```python
from build123d import *

# Parameters (mm, degrees)
F1_DEPTH  = 20
F3_DEPTH  = 25
F6_DEPTH  = 4
F8_R      = 1.395
F9_DEPTH  = 1.5
F8_R_2    = 4.25
F10_DEPTH = 112.584302492
F8_R_3    = 5.5
F11_DEPTH = 2


with BuildPart() as f1:
    # F0 (on Front) → F1 (new body)
    with BuildSketch(Plane.XZ):
        with BuildLine():
            Line((-35, 51.9615242271), (-65, 0))
            Line((-65, 0), (65, 0))
            Line((65, 0), (65, 10))
            Line((65, 10), (20.0384757729, 10))
            ThreePointArc((20.0384757729, 10), (14.8620948709, 10.6814834742), (10.0384757729, 12.6794919243))
            Line((10.0384757729, 12.6794919243), (-3.5109076373, 20.5022320835))
            ThreePointArc((-3.5109076373, 20.5022320835), (-4.2097963767, 21.4130416216), (-4.0599457429, 22.5512701892))
            Line((-4.0599457429, 22.5512701892), (-3.5599457429, 23.417295593))
            Line((-3.5599457429, 23.417295593), (-20.8804538186, 33.417295593))
            Line((-20.8804538186, 33.417295593), (-21.3804538186, 32.5512701892))
            ThreePointArc((-21.3804538186, 32.5512701892), (-22.2912633567, 31.8523814498), (-23.4294919243, 32.0022320835))
            Line((-23.4294919243, 32.0022320835), (-38.1519237886, 40.5022320835))
            ThreePointArc((-38.1519237886, 40.5022320835), (-38.8508125281, 41.4130416216), (-38.7009618943, 42.5512701892))
            Line((-38.7009618943, 42.5512701892), (-33.7009618943, 51.2115242271))
            Line((-33.7009618943, 51.2115242271), (-35, 51.9615242271))
        make_face()
        with BuildLine():
            ThreePointArc((-52.6208348754, 8.4413429511), (-54.9504640068, 11.4773747445), (-54.4509618943, 15.27146997))
            Line((-54.4509618943, 15.27146997), (-42.7009618943, 35.6230669589))
            ThreePointArc((-42.7009618943, 35.6230669589), (-39.6649301009, 37.9526960904), (-35.8708348754, 37.4531939779))
            Line((-35.8708348754, 37.4531939779), (10.2416697508, 10.8301270189))
            ThreePointArc((10.2416697508, 10.8301270189), (12.5712988822, 5.2059047745), (7.7416697508, 1.5))
            Line((7.7416697508, 1.5), (-40.5980762114, 1.5))
            Line((-40.5980762114, 1.5), (-52.6208348754, 8.4413429511))
        make_face(mode=Mode.SUBTRACT)
    extrude(amount=F1_DEPTH)

    # F2 (on face) → F3 (cut)
    with BuildSketch(Plane.XY.offset(10)):
        with BuildLine():
            Line((65, -17.963156903), (65, -15))
            Line((65, -15), (33, -15))
            ThreePointArc((33, -15), (30.8786796564, -15.8786796564), (30, -18))
            Line((30, -18), (30, -20))
            Line((30, -20), (65, -20))
            Line((65, -20), (65, -17.963156903))
        make_face()
        with BuildLine():
            Line((65, -7), (48, -7))
            ThreePointArc((48, -7), (45, -10), (48, -13))
            Line((48, -13), (65, -13))
            Line((65, -13), (65, -7))
        make_face()
        with BuildLine():
            Line((33, -5), (65, -5))
            Line((65, -5), (65, -2.036843097))
            Line((65, -2.036843097), (65, 0))
            Line((65, 0), (30, 0))
            Line((30, 0), (30, -2))
            ThreePointArc((30, -2), (30.8786796564, -4.1213203436), (33, -5))
        make_face()
    extrude(amount=-F3_DEPTH, mode=Mode.SUBTRACT)

    # F5 (on offset) → F6 (cut, through all)
    with BuildSketch(Plane(origin=(9.25, 0, 16.02146997), x_dir=(0.8660254038, 0, -0.5), z_dir=(0.5, 0, 0.8660254038))):
        with BuildLine():
            Line((-21.291651246, -6.195820753), (-28.291651246, -6.195820753))
            ThreePointArc((-28.291651246, -6.195820753), (-32.291651246, -10.195820753), (-28.291651246, -14.195820753))
            Line((-28.291651246, -14.195820753), (-21.291651246, -14.195820753))
            ThreePointArc((-21.291651246, -14.195820753), (-17.291651246, -10.195820753), (-21.291651246, -6.195820753))
        make_face()
    extrude(amount=-F6_DEPTH, mode=Mode.SUBTRACT)

    # F8 (on offset) → F9 (cut, through all)
    with BuildSketch(Plane(origin=(-48.75, 0, 28.145825623), x_dir=(0, -1, 0), z_dir=(-0.8660254038, 0, 0.5))):
        with Locations((5, -7.5)):
            Circle(F8_R)
        with Locations((5, -0.5)):
            Circle(F8_R)
        with Locations((5, 6.5)):
            Circle(F8_R)
        with Locations((15, -7.5)):
            Circle(F8_R)
        with Locations((15, -0.5)):
            Circle(F8_R)
        with Locations((15, 6.5)):
            Circle(F8_R)
    extrude(amount=-F9_DEPTH, mode=Mode.SUBTRACT)

    # F8 (on offset) → F10 (cut, through all)
    with BuildSketch(Plane(origin=(-48.75, 0, 28.145825623), x_dir=(0, -1, 0), z_dir=(-0.8660254038, 0, 0.5))):
        with Locations((10, -25)):
            Circle(F8_R_2)
    extrude(amount=-F10_DEPTH, mode=Mode.SUBTRACT)

    # F8 (on offset) → F11 (cut)
    with BuildSketch(Plane(origin=(-48.75, 0, 28.145825623), x_dir=(0, -1, 0), z_dir=(-0.8660254038, 0, 0.5))):
        with Locations((10, -25)):
            Circle(F8_R_3)
        with Locations((10, -25)):
            Circle(F8_R_2, mode=Mode.SUBTRACT)
    extrude(amount=-F11_DEPTH, mode=Mode.SUBTRACT)


solid = f1.part
```
The listing builds one solid part. Answer for the finished solid, in the listing's coordinates (mm). A direction names the side the tool comes from. Coordinates: 2 decimals unless noted, no trailing zeros. Loops run counter-clockwise (first coordinate to the right, second up) from the corner with the lowest first, then second, coordinate; pieces in that order, holes last. Notation, with made-up numbers: (31.25, 0) -> (42.25, 0) arc R32 cw to (42.25, 36) -> close; hole circle Ø10 at (68, 65.5). An arc over 180 degrees is marked (long way). Use one line per item in the form item = value. Start each with the question number.
Item 1: Flat-ended cylindrical pins translate along their axes: pin 1 Ø4 at (y, z) = (-4, 16) entering from -X; pin 2 Ø3 at (x, z) = (56, 4.5) entering from -Y; pin 3 Ø3 at (y, z) = (-12.5, 22.5) entering from +X; pin 4 Ø12 at (x, z) = (7, 23.5) entering from +Y. Find the tip coordinate at first contact, or state that the pin passes through.
Item 2: Consider L1, parallel to Y at x = 58, z = 8.5; L2, parallel to Z at x = -34, y = -17.5; L3, parallel to Z at x = 32, y = -9.5. Determine where each line is inside the solid, lowest interval first. Write a range as [from, to].
Item 3: The part is cut by section B-B on z = 45.5. Determine the outline of the cut face in (x, y), then the cut area to 3 significant figures.
Item 4: The mould has two halves that part along Z. Classify faces 5 (the face through (30.86, -4.1, 5.07)), 6 (the face through (-49.79, -9.86, 26.344)), 7 (the face through (-44.271, -5.75, 34.424)): released by +Z, released by -Z, zero draft, split by the parting line, or undercut.
Item 5: A tool of negligible diameter and unlimited length cuts with its end or side. For faces 1 (the face through (-6.71, -10.28, 22.96)), 2 (the face through (-30.7, -9.9, 36.2)), 3 (the face through (-36.236, -9.86, 46.821)), 4 (the face through (49, -5, 5)), from which of +Z, -Z, +X, -X, +Y, -Y can it reach the whole face along a straight path? Write none if from no direction.
Answer key:
q1.pin_1 = -56.92
q1.pin_2 = -15
q1.pin_3 = -3.56
q1.pin_4 = through
q2.L1 = [-15, -13], [-7, -5]
q2.L2 = [0, 1.5], [36.37, 38.11], [50.69, 51.38]
q2.L3 = [0, 10]
q3.outline = (-38.73, -20) -> (-37, -20) -> (-37, 0) -> (-38.73, 0) -> close
q3.area = 34.6 mm2
q4.face_5 = zero draft
q4.face_6 = released by +Z
q4.face_7 = undercut
q5.face_1 = +Z
q5.face_2 = +Y, -Y
q5.face_3 = +X, +Y, -Y
q5.face_4 = +Z, -Z, +X, +Y
